from build123d import *

# Parameters (mm, degrees)
SKETCH1_R           = 2.5527
SKETCH1_R_2         = 1.397
BOSS_EXTRUDE1_DEPTH = 3.175
CUT_EXTRUDE1_DEPTH  = 1.27


with BuildPart() as part:
    # Sketch1 → Boss-Extrude1 (new body)
    with BuildSketch(Plane.XY):
        with BuildLine():
            Line((16.698666352, 5.070945327), (33.168661373, 5.070945327))
            Line((33.168661373, 5.070945327), (33.168661373, -4.903410628))
            Line((33.168661373, -4.903410628), (33.168661373, -8.971340476))
            ThreePointArc((33.168661373, -8.971340476), (34.711147671, -9.490075552), (36.253633968, -8.971340476))
            Line((36.253633968, -8.971340476), (36.253633968, -4.903410628))
            Line((36.253633968, -4.903410628), (36.253633968, 5.070945327))
            Line((36.253633968, 5.070945327), (52.72362899, 5.070945327))
            Line((52.72362899, 5.070945327), (52.72362899, -33.755958849))
            Line((52.72362899, -33.755958849), (16.698666352, -33.755958849))
            Line((16.698666352, -33.755958849), (16.698666352, 5.070945327))
        make_face()
        with Locations((34.711147671, -19.07912216)):
            Circle(SKETCH1_R, mode=Mode.SUBTRACT)
        with Locations((45.918913825, -2.000621413)):
            Circle(SKETCH1_R_2, mode=Mode.SUBTRACT)
        with Locations((23.503381517, -2.000621413)):
            Circle(SKETCH1_R_2, mode=Mode.SUBTRACT)
        with Locations((23.503381517, -26.684392109)):
            Circle(SKETCH1_R_2, mode=Mode.SUBTRACT)
        with Locations((45.918913825, -26.684392109)):
            Circle(SKETCH1_R_2, mode=Mode.SUBTRACT)
    extrude(amount=BOSS_EXTRUDE1_DEPTH)

    # Sketch3 → Cut-Extrude1 (cut)
    with BuildSketch(Plane.XY.offset(3.175)):
        Polygon((40.210408985, -19.07912216), (37.460778328, -14.31662216), (31.961517014, -14.31662216), (29.211886357, -19.07912216), (31.961517014, -23.84162216), (37.460778328, -23.84162216), align=None)
    extrude(amount=-CUT_EXTRUDE1_DEPTH, mode=Mode.SUBTRACT)


solid = part.part
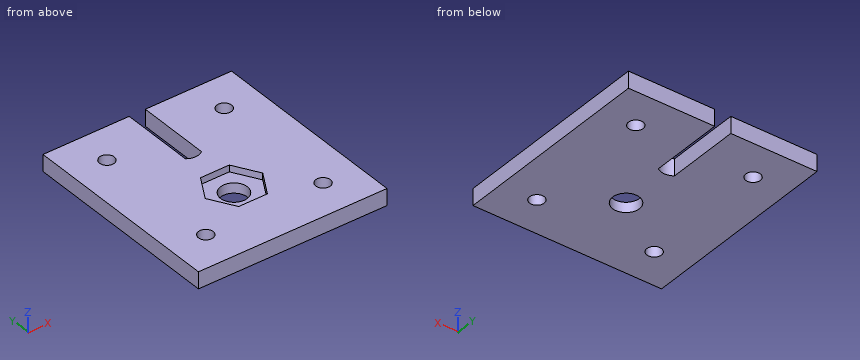
Design review of the part built by this model. Coordinates are the model's own, in mm. Round coordinates to 2 decimals unless told otherwise and drop trailing zeros. Order: outer loops, then holes, each group sorted by start corner. A loop starts at its lowest first (then second) coordinate and runs counter-clockwise, first axis right, second up.
1) Consider section A-A (y = -8.5). State the section outline as (x, z) points (3 decimals), plus the area to 3 significant figures.
The answers:
outline: (16.699, 0) - (33.169, 0) - (33.169, 3.175) - (16.699, 3.175) - close; (36.254, 0) - (52.724, 0) - (52.724, 3.175) - (36.254, 3.175) - close
area: 105 mm2
2) Consider section C-C (x = 39). State the section outline as (y, z) points (3 decimals).
The answers:
outline: (-33.756, 0) - (5.071, 0) - (5.071, 3.175) - (-16.983, 3.175) - (-16.983, 1.905) - (-21.176, 1.905) - (-21.176, 3.175) - (-33.756, 3.175) - close
3) Consider section D-D (z = 0.9). State the section outline as (x, y) points.
The answers:
outline: (16.7, -33.76) - (52.72, -33.76) - (52.72, 5.07) - (36.25, 5.07) - (36.25, -8.97) arc R2.55 cw to (33.17, -8.97) - (33.17, 5.07) - (16.7, 5.07) - close; hole circle Ø2.79 at (23.5, -26.68); hole circle Ø2.79 at (23.5, -2); hole circle Ø5.11 at (34.71, -19.08); hole circle Ø2.79 at (45.92, -26.68); hole circle Ø2.79 at (45.92, -2)
4) Consider section B-B (y = -26). State the section outline as (x, z) points (1 decimal), plus the area to 3 significant figures.
The answers:
outline: (16.7, 0) - (22.3, 0) - (22.3, 3.2) - (16.7, 3.2) - close; (24.7, 0) - (44.7, 0) - (44.7, 3.2) - (24.7, 3.2) - close; (47.1, 0) - (52.7, 0) - (52.7, 3.2) - (47.1, 3.2) - close
area: 98.9 mm2
5) For L1, parallel to Y at x = 22.5, z = 0.9; L2, parallel to X at y = -7, z = 0.25; L3, parallel to Y at x = 34.5, z = 0.95, list the stretches that pass through material, from the lowest coordinate up.
The answers:
L1: y = -33.76 to -27.66, -25.71 to -2.97, -1.03 to 5.07
L2: x = 16.7 to 33.17, 36.25 to 52.72
L3: y = -33.76 to -21.62, -16.54 to -9.48
6) Clearance check with flat-ended pins moving along their axes: pin 1 Ø6.5 at (x, y) = (34.71, -19.08) entering from +Z (3 decimals); pin 2 Ø3 at (x, y) = (36, -8) entering from -Z; pin 3 Ø2.5 at (x, y) = (23.5, -2) entering from +Z. State where each tip first meets the part, or that it passes through.
The answers:
pin 1: stops at z = 1.905
pin 2: stops at z = 0
pin 3: passes through
